Here's how the part is built. I have some questions about the finished solid (model axes, mm). A direction names the side the tool comes from. Round coordinates to 2 decimals unless told otherwise and drop trailing zeros. Order: outer loops, then holes, each group sorted by start corner. A loop starts at its lowest first (then second) coordinate and runs counter-clockwise, first axis right, second up. Notation, with made-up numbers: M 30.25,59.5 L 48.25,59.5 A20 cw 48.25,81.5 Z; hole C 66.5,7 d4. An arc over 180 degrees is marked long. Write each question's results on one line, items separated by ' | '. Start each with the question number.
Autodesk Inventor part; units mm, degrees
ref_plane "YZ Plane" through (0, 0, 0) normal (1, 0, 0) x (0, 1, 0)
ref_plane "XZ Plane" through (0, 0, 0) normal (0, 1, 0) x (-1, 0, 0)
ref_plane "XY Plane" through (0, 0, 0) normal (0, 0, 1) x (1, 0, 0)
sketch "Sketch1" plane through (0, 0, 0) normal (0, 0, 1) x (1, 0, 0)
  line L0 (0, 0) -> (25.4, 0)
  line L1 (25.4, 0) -> (25.4, 50.8)
  line L2 (25.4, 50.8) -> (0, 50.8)
  line L3 (0, 50.8) -> (0, 0)
  dimension "d0" = 25.4
  dimension "d1" = 50.8
extrude "Extrusion1" add sketch "Sketch1" along normal blind 863.6
sketch "Sketch2" plane through (0, 50.8, 0) normal (0, 1, 0) x (1, 0, 0)
  line L0 (0, -863.6) -> (25.4, -863.6)
  line L1 (25.4, 0) -> (25.4, -863.6)
  line L2 (0, 0) -> (0, -863.6)
  line L3 (0, -203.2) -> (25.4, -203.2)
  line L4 (25.4, -203.2) -> (25.4, -254)
  line L5 (25.4, -254) -> (0, -254)
  line L6 (0, -254) -> (0, -203.2)
  dimension "d5" = 50.8
  dimension "d6" = 609.6
extrude "Extrusion2" add sketch "Sketch2" along normal blind 50.8 and the other way blind 101.6 contours L2 L3 L1 L5
sketch "Sketch4" plane through (0, 50.8, 863.6) normal (0, 1, 0) x (1, 0, 0)
  line L0 (0, 609.6) -> (0, 0)
  line L1 (0, 0) -> (25.4, 0)
  line L2 (25.4, 609.6) -> (25.4, 0)
  line L3 (0, 203.2) -> (25.4, 203.2)
  line L4 (25.4, 203.2) -> (25.4, 152.4)
  line L5 (25.4, 152.4) -> (0, 152.4)
  line L6 (0, 152.4) -> (0, 203.2)
  point P0 (0, 863.6)
  dimension "d14" = 50.8
  dimension "d15" = 152.4
extrude "Extrusion4" add sketch "Sketch4" along normal blind 152.4 and the other way blind 203.2 contours L3 L2 L5 L0
shell "Shell3" thickness 3.175 removed faces 6 at (8.4667, 33.8667, 0) at (8.4667, -50.8, 220.1333) at (8.4667, 101.6, 220.1333) at (16.9333, -152.4, 694.2667) at (8.4667, 33.8667, 863.6) at (16.9333, 203.2, 694.2667)
sketch "Sketch5" plane through (25.4, 0, 0) normal (1, 0, 0) x (0, 0, -1)
  line L0 (-863.6, 50.8) -> (-863.6, 0)
  line L1 (0, 0) -> (-203.2, 0)
  line L2 (0, 0) -> (0, 50.8)
  line L3 (0, 47.625) -> (-38.1, 47.625)
  line L4 (-38.1, 47.625) -> (-38.1, 3.175)
  line L5 (-38.1, 3.175) -> (0, 3.175)
  line L6 (0, 3.175) -> (0, 47.625)
  line L7 (-863.6, 47.625) -> (-825.5, 47.625)
  line L8 (-825.5, 47.625) -> (-825.5, 3.175)
  line L9 (-825.5, 3.175) -> (-863.6, 3.175)
  line L10 (-863.6, 3.175) -> (-863.6, 47.625)
  dimension "d23" = 44.45
  dimension "d24" = 3.175
  dimension "d25" = 38.1
extrude "Extrusion5" cut sketch "Sketch5" against normal through all
sketch "Sketch6" plane through (0, 0, 0) normal (0, -1, 0) x (1, 0, 0)
  line L0 (0, 0) -> (0, 203.2)
  line L1 (0, 0) -> (25.4, 0)
  circle A0 centre (12.7, 12.7) radius 6.35
  dimension "d28" = 12.7
  dimension "d29" = 12.7
  dimension "d30" = 12.7
extrude "Extrusion6" cut sketch "Sketch6" against normal through all
sketch "Sketch7" plane through (0, 0, 863.6) normal (0, -1, 0) x (1, 0, 0)
  line L0 (25.4, -152.4) -> (25.4, 0)
  line L1 (25.4, 0) -> (0, 0)
  circle A0 centre (12.7, -12.7) radius 6.35
  point P0 (0, -863.6)
  dimension "d33" = 12.7
  dimension "d34" = 12.7
  dimension "d35" = 12.7
extrude "Extrusion7" cut sketch "Sketch7" against normal through all
sketch "Sketch8" plane through (25.4, -50.8, 254) normal (1, 0, 0) x (0, 0, -1)
  line L0 (-457.2, 254) -> (-431.8, 254)
  line L1 (-431.8, 254) -> (-431.8, 228.6)
  line L2 (-431.8, 228.6) -> (-457.2, 228.6)
  line L3 (-457.2, 228.6) -> (-457.2, 254)
  line L4 (-457.2, -101.6) -> (-431.8, -101.6)
  line L5 (-431.8, -101.6) -> (-431.8, -76.2)
  line L6 (-431.8, -76.2) -> (-457.2, -76.2)
  line L7 (-457.2, -76.2) -> (-457.2, -101.6)
  dimension "d38" = 25.4
  dimension "d39" = 25.4
extrude "Extrusion8" cut sketch "Sketch8" against normal through all
sketch "Sketch9" plane through (25.4, -50.8, 254) normal (1, 0, 0) x (0, 0, -1)
  line L0 (-431.8, 228.6) -> (-457.2, 228.6)
  line L1 (-457.2, 101.6) -> (-457.2, 228.6)
  line L2 (-457.2, -76.2) -> (-457.2, 50.8)
  line L3 (-457.2, -76.2) -> (-431.8, -76.2)
  circle A0 centre (-444.5, 203.2) radius 6.35
  circle A1 centre (-444.5, -50.8) radius 6.35
  dimension "d42" = 12.7
  dimension "d43" = 25.4
  dimension "d44" = 12.7
  dimension "d45" = 25.4
  dimension "d46" = 12.7
extrude "Extrusion9" cut sketch "Sketch9" against normal through all
sketch "Sketch10" plane through (0, 50.8, 254) normal (0, 1, 0) x (1, 0, 0)
  line L0 (0, -406.4) -> (25.4, -406.4)
  line L1 (25.4, 0) -> (25.4, -406.4)
  circle A0 centre (12.7, -368.3) radius 6.35
  point P0 (0, 254)
  dimension "d49" = 12.7
  dimension "d50" = 12.7
  dimension "d51" = 38.1
extrude "Extrusion10" cut sketch "Sketch10" against normal through all
properties part number "Frame_MainStructuralMember" material "Aluminum-6061"
(1) I want a section at A-A on z = 153. Write out the boundary of the cut face in (x, y) (3 decimals), and give its area (3 significant figures).
(2) I want a section at B-B on x = 12.7. Give the number of separate pieces and of enclosed holes in the cut face, and give its area (3 significant figures).
(3) Please list where these lines run through material, in increasing order: line 1 (Z direction, x = 4.5, y = 53) (3 decimals); line 2 (Z direction, x = 12.7, y = 48.5) (3 decimals); line 3 (Y direction, x = 0.85, z = 698.5).
(4) I'm going to push flat-ended pins straight in: pin 1 Ø2 at (x, y) = (17, -116) entering from +Z; pin 2 Ø14.5 at (x, z) = (12.7, 12.7) entering from +Y; pin 3 Ø5.5 at (x, y) = (16, -21) entering from -Z; pin 4 Ø8 at (y, z) = (46, 96) entering from -X. Where does each tip first touch, or does it pass through?
(5) If we mould it in two halves opening along Z, with no side actions, what happens to faces 6 (the flat face through (13, 50.8, 786)), 7 (the flat face through (13, 113, 711.2)), 8 (the flat face through (3.175, 26, 459))? For each: pulls with the +Z half, pulls with the -Z half, needs draft (parallel to the pull), parting line crosses it, or undercut.
(6) On a 3-axis mill with a long thin cutter (end or side, diameter ignored), from which of +Z, -Z, +X, -X, +Y, -Y can I reach the whole of each face in a straight line? I mean faces 1 (the flat face through (13, 47.625, 454)), 2 (the flat face through (13, -26, 203.2)), 3 (the flat face through (12, 177.8, 709)), 4 (the flat face through (13, 50.8, 100)), 5 (the flat face through (13, 74, 206.375)). Say none if no direction works.
Solutions:
1) outline: M 0,0 L 25.4,0 L 25.4,50.8 L 0,50.8 Z; hole M 3.175,3.175 L 22.225,3.175 L 22.225,47.625 L 3.175,47.625 Z | area: 444 mm^2
2) separate pieces: 12 | enclosed holes: 0 | area: 7,100 mm^2
3) line 1: 203.2 to 206.375, 250.825 to 254, 660.4 to 663.575, 708.025 to 711.2 | line 2: 0 to 6.35, 19.05 to 206.375, 250.825 to 615.95, 628.65 to 663.575, 708.025 to 844.55, 857.25 to 863.6 | line 3: -127 to -107.95, -95.25 to 146.05, 158.75 to 177.8
4) pin 1: z = 711.2 | pin 2: y = 50.8 | pin 3: z = 203.2 | pin 4: x = 0
5) face 6: needs draft | face 7: pulls with the +Z half | face 8: undercut
6) face 1: +Z, -Z | face 2: -Z, +X, -X, -Y | face 3: +Z, +X, -X, +Y | face 4: -Z, +X, -X, +Y | face 5: +Y, -Y
